Model file for the job. Use its own axes, mm. A direction names the side the tool comes from. Round coordinates to 2 decimals unless told otherwise and drop trailing zeros. Loops run counter-clockwise (first coordinate to the right, second up) from the corner with the lowest first, then second, coordinate; pieces in that order, holes last. Notation, with made-up numbers: (10, 36.25) - (65, 36.25) arc R13 cw to (65, 44.25) - close; hole circle Ø2 at (10.25, 37.25). An arc over 180 degrees is marked (long way). Use one line per item in the form item = value.
from build123d import *

# Parameters (mm, degrees)
SKETCH_1_R                        = 20
SKETCH_1_R_2                      = 10
EXTRUDE_1_DEPTH                   = 45
HOLE_WIZARD_M10_1_D               = 8.5
HOLE_WIZARD_M10_1_DEPTH           = 12.5
HOLE_WIZARD_M10_1_TIP             = 2.553657631
HOLE_WIZARD_M10_1_ON_FACE_2_D     = 8.5
HOLE_WIZARD_M10_1_ON_FACE_2_DEPTH = 12.5
HOLE_WIZARD_M10_1_ON_FACE_2_TIP   = 2.553657631
SKETCH_4_R                        = 20
SKETCH_4_R_2                      = 10
EXTRUDE_2_DEPTH                   = 105
EXTRUDE_START                     = -5
SKETCH_5_R                        = 28.4
SKETCH_5_R_2                      = 20
EXTRUDE_3_DEPTH                   = 5
HOLE_WIZARD_4_0_4_1_D             = 4
CUT_EXTRUDE_2_DEPTH               = 25


with BuildPart() as part:
    # Sketch 1 → Extrude 1 (new body)
    with BuildSketch(Plane(origin=(0, 0, 0), x_dir=(1, 0, 0), z_dir=(0, 1, 0))):
        with Locations(Location((0, 0, 0), (0, 0, 90))):
            Circle(SKETCH_1_R)
        with Locations(Location((0, 0, 0), (0, 0, 90))):
            Circle(SKETCH_1_R_2, mode=Mode.SUBTRACT)
    extrude(amount=EXTRUDE_1_DEPTH)

    # Hole Wizard M10 _1
    with Locations(Plane(origin=(0, 22.5, -20), x_dir=(0, -1, 0), z_dir=(0, 0, -1))):
        with Locations((0, 0)):
            Hole(HOLE_WIZARD_M10_1_D / 2, depth=HOLE_WIZARD_M10_1_DEPTH)
            with Locations((0, 0, -(HOLE_WIZARD_M10_1_DEPTH + HOLE_WIZARD_M10_1_TIP / 2))):  # 118° drill point
                Cone(0, HOLE_WIZARD_M10_1_D / 2, HOLE_WIZARD_M10_1_TIP, mode=Mode.SUBTRACT)

    # Hole Wizard M10 _1 on face 2
    with Locations(Plane(origin=(0, 22.5, 20), x_dir=(1, 0, 0), z_dir=(0, 0, 1))):
        with Locations((0, 0)):
            Hole(HOLE_WIZARD_M10_1_ON_FACE_2_D / 2, depth=HOLE_WIZARD_M10_1_ON_FACE_2_DEPTH)
            with Locations((0, 0, -(HOLE_WIZARD_M10_1_ON_FACE_2_DEPTH + HOLE_WIZARD_M10_1_ON_FACE_2_TIP / 2))):  # 118° drill point
                Cone(0, HOLE_WIZARD_M10_1_ON_FACE_2_D / 2, HOLE_WIZARD_M10_1_ON_FACE_2_TIP, mode=Mode.SUBTRACT)

    # Sketch 4 → Extrude 2 (add)
    with BuildSketch(Plane(origin=(0, 45, 0), x_dir=(1, 0, 0), z_dir=(0, 1, 0))):
        with Locations(Location((0, 0, 0), (0, 0, 270))):
            Circle(SKETCH_4_R)
        with Locations(Location((0, 0, 0), (0, 0, 270))):
            Circle(SKETCH_4_R_2, mode=Mode.SUBTRACT)
    extrude(amount=EXTRUDE_2_DEPTH)

    # Sketch 5 → Extrude 3 (add)
    with BuildSketch(Plane(origin=(0, 150, 0), x_dir=(1, 0, 0), z_dir=(0, 1, 0)).offset(EXTRUDE_START)):
        with Locations(Location((0, 0, 0), (0, 0, 270))):
            Circle(SKETCH_5_R)
        with Locations(Location((0, 0, 0), (0, 0, 270))):
            Circle(SKETCH_5_R_2, mode=Mode.SUBTRACT)
    extrude(amount=EXTRUDE_3_DEPTH)

    # Hole Wizard 4.0 _4_ _1 (through all)
    with Locations(Plane.XZ.offset(-145)):
        with Locations((-18.03122292, -18.03122292), (-18.03122292, 18.03122292), (18.03122292, 18.03122292), (18.03122292, -18.03122292)):
            Hole(HOLE_WIZARD_4_0_4_1_D / 2)

    # Sketch 10 → Cut-Extrude 2 (cut)
    with BuildSketch(Plane.XY):
        Polygon((0, 120), (8, 120), (8, 110), (-8, 110), (-8, 120), align=None)
    extrude(amount=CUT_EXTRUDE_2_DEPTH, mode=Mode.SUBTRACT)


solid = part.part
1. Tool access for faces 1 (the flat face through (17, 145, -11)), 2 (the flat face through (-8, 115, 12)), 3 (the cylindrical face through (-19.106, 147.535, 19.718)): list every direction of +Z, -Z, +X, -X, +Y, -Y with a clear straight run to the whole face (end or side of a thin tool).
Geometry check:
face_1 = -Y
face_2 = +Z
face_3 = +Y, -Y
2. Cut at A-A, the plane x = 0. Give the cut face in (y, z), plus the area to 3 significant figures.
Geometry check:
outline = (0, -20) - (18.25, -20) - (18.25, -10) - (0, -10) - close; (0, 10) - (18.25, 10) - (18.25, 20) - (0, 20) - close; (26.75, -20) - (145, -20) - (145, -28.4) - (150, -28.4) - (150, -10) - (26.75, -10) - close; (26.75, 10) - (110, 10) - (110, 20) - (26.75, 20) - close; (120, 10) - (150, 10) - (150, 28.4) - (145, 28.4) - (145, 20) - (120, 20) - close
area = 2,810 mm^2
3. Pull direction X, two halves, no side cores. Call faces 4 (the flat face through (-9, 0, 5)), 5 (the cylindrical face through (23.947, 147.465, 15.268)), 6 (the flat face through (0, 110, 14)): +X half, -X half, draft (parallel to the pull), parting line (faces both ways), or undercut.
Geometry check:
face_4 = draft
face_5 = parting line
face_6 = undercut
4. Flat gauge pins, fed straight in: pin 1 (8 mm diameter, centred on x = -5.5, y = 23.5, fed in from -Z); pin 2 (2.5 mm diameter, centred on x = -18.03, z = 18.03, fed in from -Y); pin 3 (5 mm diameter, centred on x = 18.03, z = 18.03, fed in from -Y); pin 4 (12 mm diameter, centred on y = 115, z = -3, fed in from +X). Where does each tip first touch, or does it go through?
Geometry check:
pin_1 = -19.86
pin_2 = through
pin_3 = 145
pin_4 = 20
5. Cut at D-D, the plane z = 11.5. Give the cut face in (x, y).
Geometry check:
outline = (-25.97, 145) - (-16.36, 145) - (-16.36, 0) - (16.36, 0) - (16.36, 145) - (25.97, 145) - (25.97, 150) - (-25.97, 150) - close; hole (-8, 110) - (8, 110) - (8, 120) - (-8, 120) - close; hole circle Ø8.5 at (0, 22.5)
6. Wall check: probe 1 along X at (y, z) = (117.5, -3); probe 2 along X at (y, z) = (22, -15); probe 3 along Z at (x, y) = (5, 131.5). Give the ranges that are in metal, low to high.
Geometry check:
probe_1 = -19.77 to -9.54, 9.54 to 19.77
probe_2 = -13.23 to -4.22, 4.22 to 13.23
probe_3 = -19.36 to -8.66, 8.66 to 19.36
7. Cut at B-B, the plane z = 0. Give the cut face in (x, y).
Geometry check:
outline = (-28.4, 145) - (-20, 145) - (-20, 0) - (-10, 0) - (-10, 150) - (-28.4, 150) - close; (10, 0) - (20, 0) - (20, 145) - (28.4, 145) - (28.4, 150) - (10, 150) - close
8. Cut at C-C, the plane y = 22.5. Give the cut face in (x, z).
Geometry check:
outline = (-4.25, -19.54) - (-4.25, -9.05) arc R10 cw to (-4.25, 9.05) - (-4.25, 19.54) arc R20 ccw to start; (4.25, -19.54) arc R20 ccw to (4.25, 19.54) - (4.25, 9.05) arc R10 cw to (4.25, -9.05) - close
